from build123d import *

# Parameters (mm, degrees)
BOSS_EXTRUDE1_DEPTH = 15.9
FILLET1_R           = 1.6


with BuildPart() as part:
    # BodySke → Base-Revolve (revolve)
    with BuildSketch(Plane.XY, mode=Mode.PRIVATE) as base_revolve_sk:
        with BuildLine():
            Line((9.0906, 23), (10.9, 23))
            Line((10.9, 23), (10.9, 10))
            Line((10.9, 10), (89.526, 10))
            Line((89.526, 10), (90.9, 8.626))
            Line((90.9, 8.626), (90.9, 0))
            Line((90.9, 0), (0, 0))
            ThreePointArc((0, 0), (2.355084776, 12.365668283), (9.0906, 23))
        make_face()
    revolve(base_revolve_sk.sketch.rotate(Axis((-31.75, 0, 0), (1, 0, 0)), 90), axis=Axis((-31.75, 0, 0), (1, 0, 0)))

    # Sketch1 → Boss-Extrude1 (add)
    with BuildSketch(Plane(origin=(10.9, 0, 0), x_dir=(0, 0, -1), z_dir=(1, 0, 0))):
        Polygon((0, 14.142135624), (14.142135624, 0), (0, -14.142135624), (-14.142135624, 0), align=None)
    extrude(amount=BOSS_EXTRUDE1_DEPTH)

    # Sketch2 → Cut-Revolve1 (revolve, cut)
    with BuildSketch(Plane.XY):
        Polygon((26.8, 10), (31.8, 10), (31.8, 24), (12.8, 24), align=None)
    revolve(axis=Axis((0, 0, 0), (1, 0, 0)), mode=Mode.SUBTRACT)

    # Fillet1
    fillet1_edges = [part.edges().sort_by_distance(p)[0] for p in [
        (10.9, 7.071067812, -7.071067812),
        (10.9, -7.071067812, -7.071067812),
        (10.9, 7.071067812, 7.071067812),
        (10.9, -7.071067812, 7.071067812),
    ]]
    fillet(fillet1_edges, radius=FILLET1_R)


solid = part.part
The model under review builds one solid part; all positions refer to its coordinate system, in mm. A direction names the side the tool comes from. Round coordinates to 2 decimals unless told otherwise and drop trailing zeros. Order: outer loops, then holes, each group sorted by start corner. A loop starts at its lowest first (then second) coordinate and runs counter-clockwise, first axis right, second up. Notation, with made-up numbers: (-35, 17) -> (-10, 17) arc R29 cw to (-10, 38) -> close; hole circle Ø10 at (-31, 25). An arc over 180 degrees is marked (long way). Write item = value, one per line. Start each with the question number.
Item 1: Consider section C-C on x = 37. Write out the cut boundary in (y, z).
Item 2: For faces 1 (the face through (19.55, -6.97, -7.17)), 2 (the face through (19.55, -7.17, 6.97)), 3 (the face through (10.9, 10, 10)), list the 3-axis set-ups (+Z, -Z, +X, -X, +Y, -Y) from which the entire face can be reached by the end or side of a thin tool; tool diameter is ignored.
Item 3: For line 1 along Z through (x, y) = (77, 0.5); line 2 along X through (y, z) = (-9, 19); line 3 along Z through (x, y) = (31, 6), list the stretches that pass through material, from the lowest coordinate up.
Item 4: Consider section B-B on y = -18. Write out the cut boundary in (x, z), plus the area to 3 significant figures.
Item 5: Clearance check with flat-ended pins moving along their axes: pin 1 Ø10 at (x, z) = (16, -9.5) entering from +Y; pin 2 Ø1.5 at (x, y) = (19, -2) entering from -Z; pin 3 Ø8 at (y, z) = (0.5, -17) entering from -X. State where each tip first meets the part, or that it passes through.
Item 6: Consider section A-A on x = 15. Write out the cut boundary in (y, z).
Conclusion:
q1.outline = circle Ø20 at (0, 0)
q2.face_1 = -Z, +X, -Y
q2.face_2 = +Z, +X, -Y
q2.face_3 = +X
q3.line_1 = -9.99 to 9.99
q3.line_2 = 7.38 to 10.9
q3.line_3 = -8 to 8
q4.outline = (9.09, -14.32) -> (10.9, -14.32) -> (10.9, 14.32) -> (9.09, 14.32) arc R28.42 ccw to start
q4.area = 127 mm2
q5.pin_1 = 9.64
q5.pin_2 = -12.89
q5.pin_3 = 2.62
q6.outline = (-14.14, 0) -> (0, -14.14) -> (14.14, 0) -> (0, 14.14) -> close
